The listing builds one solid part. Answer for the finished solid, in the listing's coordinates (mm). A direction names the side the tool comes from. Coordinates: 2 decimals unless noted, no trailing zeros. Order: outer loops, then holes, each group sorted by start corner. A loop starts at its lowest first (then second) coordinate and runs counter-clockwise, first axis right, second up.
```python
from build123d import *

# Parameters (mm, degrees)
SKETCH2_W          = 469.9
SKETCH2_H          = 63.5
EXTRUDE1_DEPTH     = 17.78
SKETCH3_W          = 17.78
SKETCH3_H          = 63.5
CUT_EXTRUDE1_DEPTH = 5.08
SKETCH4_R          = 1.5875
CUT_EXTRUDE2_DEPTH = 17.78
SKETCH5_R          = 1.5875
CUT_EXTRUDE3_DEPTH = 17.78


with BuildPart() as part:
    # Sketch2 → Extrude1 (new body)
    with BuildSketch(Plane.XY):
        with Locations((11073.341666666, -5688.0125)):
            Rectangle(SKETCH2_W, SKETCH2_H)
    extrude(amount=-EXTRUDE1_DEPTH)

    # Sketch3 → Cut-Extrude1 (cut)
    with BuildSketch(Plane.XY):
        with Locations((11299.401666666, -5688.0125)):
            Rectangle(SKETCH3_W, SKETCH3_H)
        with Locations((10847.281666666, -5688.0125)):
            Rectangle(SKETCH3_W, SKETCH3_H)
    extrude(amount=-CUT_EXTRUDE1_DEPTH, mode=Mode.SUBTRACT)

    # Sketch4 → Cut-Extrude2 (cut)
    with BuildSketch(Plane.XY):
        with Locations((10847.281666666, -5668.9625)):
            Circle(SKETCH4_R)
        with Locations((10847.281666666, -5707.0625)):
            Circle(SKETCH4_R)
        with Locations((11299.401666666, -5707.0625)):
            Circle(SKETCH4_R)
        with Locations((11299.401666666, -5668.9625)):
            Circle(SKETCH4_R)
    extrude(amount=-CUT_EXTRUDE2_DEPTH, mode=Mode.SUBTRACT)

    # Sketch5 → Cut-Extrude3 (cut)
    with BuildSketch(Plane(origin=(0, 0, -17.78), x_dir=(-1, 0, 0), z_dir=(0, 0, -1))):
        with Locations((-10911.416666665, -5690.78745)):
            Circle(SKETCH5_R)
        with Locations((-10962.216666665, -5690.78745)):
            Circle(SKETCH5_R)
        with Locations((-11254.316666665, -5690.78745)):
            Circle(SKETCH5_R)
        with Locations((-11305.116666665, -5690.78745)):
            Circle(SKETCH5_R)
    extrude(amount=-CUT_EXTRUDE3_DEPTH, mode=Mode.SUBTRACT)


solid = part.part
```
1) A cutting plane is placed at A-A, the plane y = -5663.5. Write down the section's boundary in (x, z).
2) Each of these flat-tipped pins is pushed along its axis until it touches: P1, Ø9, axis at x = 11300, y = -5677, coming from the +Z side; P2, Ø2, axis at y = -5672, z = -2.5, coming from the -X side; P3, Ø5, axis at x = 11299.4, y = -5707.06, coming from the -Z side; P4, Ø1.5, axis at y = -5692, z = -2.5, coming from the +X side. Where does it stop, or does it pass through?
3) Straight lines are drawn through the part: probe 1 along X at (y, z) = (-5669, -8.25); probe 2 along X at (y, z) = (-5668, -9.25); probe 3 along X at (y, z) = (-5667.5, -4.25). For each, find the intervals that lie inside material, in ascending order.
4) For faces 1 (the flat face through (11299, -5688, -5.08)), 2 (the flat face through (11070, -5656.262, -9)), 3 (the flat face through (10847, -5688, -5.08)), determine the directions among +Z, -Z, +X, -X, +Y, -Y from which every point of the face is accessible in a straight line to the end or side of a thin tool.
Working result:
1. outline: (10838.39, -17.78) - (11308.29, -17.78) - (11308.29, -5.08) - (11290.51, -5.08) - (11290.51, 0) - (10856.17, 0) - (10856.17, -5.08) - (10838.39, -5.08) - close
2. P1: stops at z = -5.08
2. P2: stops at x = 10856.17
2. P3: stops at z = -17.78
2. P4: stops at x = 11290.51
3. probe 1: x = 10838.39 to 10845.69, 10848.87 to 11297.81, 11300.99 to 11308.29
3. probe 2: x = 10838.39 to 10846.02, 10848.54 to 11298.14, 11300.66 to 11308.29
3. probe 3: x = 10856.17 to 11290.51
4. face 1: +Z, +X, +Y, -Y
4. face 2: +Z, -Z, +X, -X, +Y
4. face 3: +Z, -X, +Y, -Y
